Autodesk Inventor part; units mm, degrees
ref_plane "YZ Plane" through (0, 0, 0) normal (1, 0, 0) x (0, 1, 0)
ref_plane "XZ Plane" through (0, 0, 0) normal (0, 1, 0) x (-1, 0, 0)
ref_plane "XY Plane" through (0, 0, 0) normal (0, 0, 1) x (1, 0, 0)
sketch "Sketch1" plane through (0, 0, 0) normal (0, 0, 1) x (1, 0, 0)
  line L0 (-3.4123, 0.1305) -> (6.0877, 0.1305)
  line L1 (6.0877, 0.1305) -> (6.0877, -2.4395)
  line L2 (6.0877, -2.4395) -> (-3.4123, -2.4395)
  line L3 (-3.4123, -2.4395) -> (-3.4123, 0.1305)
  circle A0 centre (-2.1273, -1.1545) radius 1.285
  circle A1 centre (4.8027, -1.1545) radius 1.285
  line L4 (-4.6123, 1.5305) -> (7.2877, 1.5305)
  line L5 (7.2877, 1.5305) -> (7.2877, -2.4395)
  line L6 (7.2877, -2.4395) -> (-4.6123, -2.4395)
  line L7 (-4.6123, -2.4395) -> (-4.6123, 1.5305)
  point P0 (0, 0)
  point P1 (-3.4123, -2.4395)
  point P2 (-3.4123, -1.1545)
  point P3 (-2.1273, 0.1305)
  point P4 (4.8027, 0.1305)
  point P5 (6.0877, -1.1545)
  point P6 (6.0877, -2.4395)
  point P7 (4.8027, -2.4395)
  point P8 (-2.1273, -2.4395)
  dimension "d0" = 2.57
  dimension "d1" = 9.5
  dimension "d2" = 1.285
  dimension "d3" = 1.285
  dimension "d4" = 1.2
  dimension "d5" = 1.2
  dimension "d6" = 1.4
extrude "Extrusion1" add sketch "Sketch1" along normal blind 4 contours L3 L6 L7 L4 L5 L1 L0 | L0 A0 L3 | L0 L1 A1
sketch "Sketch2" plane through (0, 0, 0) normal (0, 0, -1) x (-1, 0, 0)
  line L0 (-6.0877, -2.4395) -> (-7.2877, -2.4395)
  line L1 (-11.0877, 6.1305) -> (-6.6877, 6.1305)
  line L2 (-6.6877, 6.1305) -> (-6.6877, -2.4395)
  line L3 (-6.6877, -2.4395) -> (-11.0877, -2.4395)
  line L4 (-11.0877, -2.4395) -> (-11.0877, 6.1305)
  line L5 (4.6123, -2.4395) -> (3.4123, -2.4395)
  line L6 (4.0123, -2.4395) -> (9.4123, -2.4395)
  line L7 (9.4123, -2.4395) -> (9.4123, 6.1305)
  line L8 (9.4123, 6.1305) -> (4.0123, 6.1305)
  line L9 (4.0123, 6.1305) -> (4.0123, -2.4395)
  line L10 (-7.2877, 1.5305) -> (4.6123, 1.5305)
  line L11 (-6.6877, 6.1305) -> (4.0123, 6.1305)
  line L12 (4.0123, 6.1305) -> (4.0123, 1.5305)
  line L13 (4.0123, 1.5305) -> (-6.6877, 1.5305)
  line L14 (-6.6877, 1.5305) -> (-6.6877, 6.1305)
  line L15 (-6.0877, -1.1545) -> (-6.0877, -2.4395)
  line L16 (3.4123, -2.4395) -> (3.4123, -1.1545)
  line L17 (2.1273, 0.1305) -> (-4.8027, 0.1305)
  point P0 (0, 0)
  point P1 (-6.6877, 1.5305)
  point P2 (4.6123, -2.4395)
  dimension "d9" = 5
  dimension "d10" = 6
  dimension "d11" = 6
extrude "Extrusion2" add sketch "Sketch2" against normal blind 1.2
fillet "Fillet1" radius 2.6 2 edges at (-4.6123, 1.5305, 2.6) (7.2877, 1.5305, 2.6)
sketch "Sketch3" plane through (-4.6123, -2.4395, 4) normal (0, -1, 0) x (1, 0, 0)
  line L0 (15.7, -2.8) -> (-4.8, -2.8)
  line L1 (1.2, -4) -> (1.2, 0)
  line L2 (-4.8, -2.8) -> (1.2, -2.8)
  line L3 (1.2, -2.8) -> (1.2, -4)
  line L4 (1.2, -4) -> (-4.8, -4)
  line L5 (-4.8, -4) -> (-4.8, -2.8)
  line L6 (0, -2.8) -> (0, 0)
  line L7 (0, 0) -> (1.2, 0)
  line L8 (1.2, 0) -> (1.2, -2.8)
  line L9 (1.2, -2.8) -> (0, -2.8)
  line L10 (0, -2.8) -> (0, 0)
  line L11 (11.9, -2.8) -> (11.9, 0)
  line L12 (10.7, -4) -> (10.7, 0)
  line L13 (11.9, 0) -> (10.7, 0)
  line L14 (10.7, 0) -> (10.7, -2.8)
  line L15 (10.7, -2.8) -> (11.9, -2.8)
  line L16 (11.9, -2.8) -> (11.9, 0)
  line L17 (15.7, -2.8) -> (10.7, -2.8)
  line L18 (10.7, -2.8) -> (10.7, -4)
  line L19 (10.7, -4) -> (15.7, -4)
  line L20 (15.7, -4) -> (15.7, -2.8)
  point P0 (4.6123, -4)
  point P1 (1.2, 0)
extrude "Extrusion3" add sketch "Sketch3" along normal blind 1.6
fillet "Fillet2" radius 0.6 5 edges at (6.5262, 0.769, 1.2) (1.3377, 1.5305, 1.2) (-3.8507, 0.769, 1.2) (-4.6123, -2.5545, 1.2) (7.2877, -2.5545, 1.2)
fillet "Fillet3" radius 1 4 edges at (-9.4123, -4.0395, 0.6) (-9.4123, 6.1305, 0.6) (11.0877, 6.1305, 0.6) (11.0877, -4.0395, 0.6)
properties part number "charge_support"
Check sheet for the modelled part. Datum: model origin and axes. Units: mm. A direction names the side the tool comes from. Round coordinates to 2 decimals unless told otherwise and drop trailing zeros. Order: outer loops, then holes, each group sorted by start corner. A loop starts at its lowest first (then second) coordinate and runs counter-clockwise, first axis right, second up.
1) Section check D-D (y = 4.5). Record the boundary of the cut face in (x, z).
2) Tool access check on faces 4 (the cylindrical face through (6.546, 0.749, 2.915)), 5 (the flat face through (-4.612, -3, 3)), 6 (the flat face through (6.088, -3, 2)), 7 (the flat face through (1, 3, 1.2)). Record the directions out of +Z, -Z, +X, -X, +Y, -Y that give a thin tool (end or side, any length) a straight path to the whole face; none if there is none.
3) Mould release check, pull along X, two halves, no side actions. Record for faces 1 (the flat face through (-9.412, 1, 1)), 2 (the flat face through (-3.412, -3, 2)), 3 (the flat face through (1, 2, 0)): +X half, -X half, draft (parallel to the pull), parting line (faces both ways), or undercut.
4) Section check A-A (y = -2.5). Record the boundary of the cut face in (x, z), and give its area (3 significant figures).
5) Section check C-C (x = -1.5). Record the boundary of the cut face in (y, z).
6) Go/stop test with flat-tipped pins: pin 1 Ø1.1 at (x, z) = (2, 3) entering from +Y; pin 2 Ø1 at (x, y) = (-2, -1.5) entering from +Z; pin 3 Ø0.9 at (y, z) = (-3, 3) entering from +X; pin 4 Ø0.9 at (y, z) = (-2.5, 2.5) entering from -X. Record where each tip stops, or that it passes through.
7) Section check B-B (z = 0.9). Record the boundary of the cut face in (x, y) (1 decimal), and give its area (3 significant figures).
8) Scan lines: line 1 (X direction, y = -1.5, z = 3.7); line 2 (X direction, y = -2.25, z = 1.15); line 3 (Y direction, x = -1.25, z = 2.3). Record each from-to range of solid material in increasing order.
Result:
1. outline: (-9.41, 0) - (11.09, 0) - (11.09, 1.2) - (-9.41, 1.2) - close
2. face 4: +Z, +X, +Y
2. face 5: +Z, -X, +Y, -Y
2. face 6: +Z, -Z, -Y
2. face 7: +Z, +Y
3. face 1: -X half
3. face 2: undercut
3. face 3: draft
4. outline: (-9.41, 0) - (-3.41, 0) - (-3.41, 4) - (-4.61, 4) - (-4.61, 1.8) arc R0.6 cw to (-5.21, 1.2) - (-9.41, 1.2) - close; (6.09, 0) - (11.09, 0) - (11.09, 1.2) - (7.89, 1.2) arc R0.6 cw to (7.29, 1.8) - (7.29, 4) - (6.09, 4) - close
4. area: 20.1 mm2
5. outline: (0.13, 0) - (6.13, 0) - (6.13, 1.2) - (2.13, 1.2) arc R0.6 cw to (1.53, 1.8) - (1.53, 4) - (0.13, 4) - close
6. pin 1: stops at y = 1.53
6. pin 2: passes through
6. pin 3: stops at x = 7.29
6. pin 4: stops at x = -4.61
7. outline: (-9.4, -3) arc R1 ccw to (-8.4, -4) - (-3.4, -4) - (-3.4, -1.2) arc R1.3 cw to (-2.1, 0.1) - (4.8, 0.1) arc R1.3 cw to (6.1, -1.2) - (6.1, -4) - (10.1, -4) arc R1 ccw to (11.1, -3) - (11.1, 5.1) arc R1 ccw to (10.1, 6.1) - (-8.4, 6.1) arc R1 ccw to (-9.4, 5.1) - close
7. area: 169 mm2
8. line 1: x = -4.61 to -3.41, 6.09 to 7.29
8. line 2: x = -9.41 to -3.41, 6.09 to 11.09
8. line 3: y = 0.13 to 1.53
